```python
from build123d import *

# Parameters (mm, degrees)
F0_W     = 152.4
F0_H     = 114.3
F1_DEPTH = 6.35
F3_DEPTH = 38.1


with BuildPart() as f1:
    # F0 (on Top) → F1 (new body, symmetric)
    with BuildSketch(Plane.XY):
        with Locations((-76.2, 57.15)):
            Rectangle(F0_W, F0_H)
    extrude(amount=F1_DEPTH, both=True)

    # F2 (on face) → F3 (join)
    with BuildSketch(Plane.XY.offset(6.35)):
        Polygon((-53.5205122421, 97.79), (-116.84, 34.4705122421), (-107.8597438789, 25.4902561211), (-98.8794877579, 16.51), (-35.56, 79.8294877579), (-44.5402561211, 88.8097438789), align=None)
        with BuildLine():
            Line((-107.8597438789, 25.4902561211), (-116.84, 34.4705122421))
            ThreePointArc((-116.84, 34.4705122421), (-116.84, 16.51), (-98.8794877579, 16.51))
            Line((-98.8794877579, 16.51), (-107.8597438789, 25.4902561211))
        make_face()
        with BuildLine():
            ThreePointArc((-35.56, 79.8294877579), (-35.56, 97.79), (-53.5205122421, 97.79))
            Line((-53.5205122421, 97.79), (-44.5402561211, 88.8097438789))
            Line((-44.5402561211, 88.8097438789), (-35.56, 79.8294877579))
        make_face()
    extrude(amount=F3_DEPTH)


solid = f1.part
```
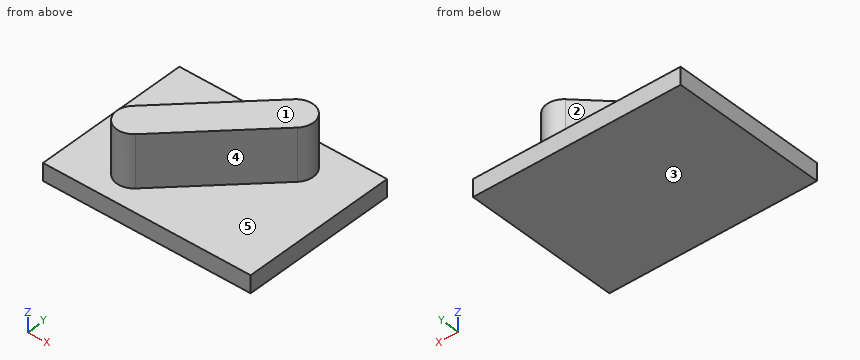
Build history of the part. All positions in model axes, mm. Face numbers are marked on the shaded views. A direction names the side the tool comes from. Coordinates: 2 decimals unless noted, no trailing zeros. Order: outer loops, then holes, each group sorted by start corner. A loop starts at its lowest first (then second) coordinate and runs counter-clockwise, first axis right, second up.
Item 1: Saw through at C-C on z = 29.5. List the corners of the cut face in (x, y), then the cut area to 3 significant figures.
Filled in:
outline: (-116.84, 34.47) arc R12.7 ccw to (-98.88, 16.51) - (-35.56, 79.83) arc R12.7 ccw to (-53.52, 97.79) - close
area: 2,780 mm2
Item 2: Saw through at A-A on y = 69.5. List the corners of the cut face in (x, z), then the cut area to 3 significant figures.
Filled in:
outline: (-152.4, -6.35) - (0, -6.35) - (0, 6.35) - (-45.89, 6.35) - (-45.89, 44.45) - (-81.81, 44.45) - (-81.81, 6.35) - (-152.4, 6.35) - close
area: 3,300 mm2
Item 3: Saw through at D-D on x = -139. List the corners of the cut face in (y, z), then the cut area to 3 significant figures.
Filled in:
outline: (0, -6.35) - (114.3, -6.35) - (114.3, 6.35) - (0, 6.35) - close
area: 1,450 mm2
Item 4: Tool access for the marked faces 1, 2, 3, 4 and 5: list every direction of +Z, -Z, +X, -X, +Y, -Y with a clear straight run to the whole face (end or side of a thin tool).
Filled in:
face 1: +Z, +X, -X, +Y, -Y
face 2: +Z, -X, +Y
face 3: -Z, +X, -X, +Y, -Y
face 4: +Z, +X, -Y
face 5: +Z
Item 5: Drill centre lines: L1, parallel to Z at x = -21.5, y = 103.5; L2, parallel to X at y = 63, z = 7; L3, parallel to Y at x = -61.5, z = 27. Where is each one in solid material? Low to high.
Filled in:
L1: z = -6.35 to 6.35
L2: x = -88.31 to -52.39
L3: y = 53.89 to 89.81
Item 6: Saw through at B-B on x = -114.5. List the corners of the cut face in (y, z), then the cut area to 3 significant figures.
Filled in:
outline: (0, -6.35) - (114.3, -6.35) - (114.3, 6.35) - (36.81, 6.35) - (36.81, 44.45) - (14.66, 44.45) - (14.66, 6.35) - (0, 6.35) - close
area: 2,300 mm2
Item 7: Drop flat-ended pins along their axis: pin 1 Ø3 at (x, z) = (-117, 12.5) entering from +Y; pin 2 Ø5 at (y, z) = (53, 19) entering from +X; pin 3 Ø5 at (x, y) = (-57, 26.5) entering from +Z. Give the stop position or say it passes through.
Filled in:
pin 1: stops at y = 35.81
pin 2: stops at x = -59.89
pin 3: stops at z = 6.35
